from build123d import *

# Parameters (mm, degrees)
EXTRU_MINCE1_DEPTH         = 100
EXTRU_MINCE2_DEPTH         = 5
EXTRU_MINCE3_DEPTH         = 5
CONG_1_R                   = 10
R_P_TITION_START           = 80
R_P_TITION_LIN_AIRE1_DEPTH = 5
CONG_2_R                   = 5


# Read off the part's stored shape, not the designer's step: Répétition linéaire1
with BuildPart() as part:
    # Esquisse1 → Extru.-Mince1 (new body)
    with BuildSketch(Plane.XY):
        Polygon((0, 0), (-65.404068622, 0), (-4.782306964, 200), (-0.954292763, 198.839695178), (-60.011920576, 4), (0, 4), align=None)
    extrude(amount=EXTRU_MINCE1_DEPTH)

    # Esquisse2 → Extru.-Mince2 (add)
    with BuildSketch(Plane.XY.offset(10)):
        Polygon((-11.060818094, 179.286279518), (-14.23934022, 192.904801434), (-10.344030265, 193.813955082), (-7.16550814, 180.195433166), align=None)
        Polygon((-40.068438655, 83.585924506), (-43.246960781, 97.204446422), (-39.351650826, 98.11360007), (-36.1731287, 84.495078154), align=None)
    extrude(amount=EXTRU_MINCE2_DEPTH)

    # Esquisse3 → Extru.-Mince3 (add)
    with BuildSketch(Plane.XY.offset(45)):
        Polygon((-18.341466727, 155.266361808), (-26.702263311, 169.885700914), (-23.229995746, 171.871489915), (-14.869199162, 157.252150809), align=None)
        Polygon((-32.333054107, 109.106082076), (-40.693850691, 123.725421182), (-37.221583126, 125.711210183), (-28.860786542, 111.091871077), align=None)
        Polygon((-51.073031786, 47.280172809), (-59.433828371, 61.899511915), (-55.961560806, 63.885300916), (-47.600764221, 49.26596181), align=None)
    extrude(amount=EXTRU_MINCE3_DEPTH)

    # Congé1
    cong_1_edges = [part.edges().sort_by_distance(p)[0] for p in [
        (-11.060818094, 179.286279518, 12.5),
        (-40.068438655, 83.585924506, 12.5),
        (-18.341466727, 155.266361808, 47.5),
        (-32.333054107, 109.106082076, 47.5),
        (-51.073031786, 47.280172809, 47.5),
    ]]
    fillet(cong_1_edges, radius=CONG_1_R)

    # Répétition linéaire1 outline → Répétition linéaire1 (add)
    with BuildSketch(Plane.XY.offset(R_P_TITION_START)):
        with BuildLine():
            Line((-40.845695505, 81.021641222), (-37.74782901, 91.241952907))
            Line((-37.74782901, 91.241952907), (-39.351650826, 98.11360007))
            Line((-39.351650826, 98.11360007), (-43.246960781, 97.204446422))
            Line((-43.246960781, 97.204446422), (-40.677456119, 86.195287398))
            ThreePointArc((-40.677456119, 86.195287398), (-40.421014092, 83.597389742), (-40.845695505, 81.021641222))
        make_face()
        with BuildLine():
            Line((-8.74020845, 186.942307919), (-10.344030265, 193.813955082))
            Line((-10.344030265, 193.813955082), (-14.23934022, 192.904801434))
            Line((-14.23934022, 192.904801434), (-11.669835559, 181.89564241))
            ThreePointArc((-11.669835559, 181.89564241), (-11.413393531, 179.297744754), (-11.838074945, 176.721996234))
            Line((-11.838074945, 176.721996234), (-8.74020845, 186.942307919))
        make_face()
    extrude(amount=R_P_TITION_LIN_AIRE1_DEPTH)

    # Congé2
    cong_2_edges = [part.edges().sort_by_distance(p)[0] for p in [
        (0, 2, 100),
        (0, 2, 0),
        (-2.868299864, 199.419847589, 0),
        (-2.868299864, 199.419847589, 100),
        (-60.011920576, 4, 50),
        (-65.404068622, 0, 50),
    ]]
    fillet(cong_2_edges, radius=CONG_2_R)


solid = part.part
Source: CAD feature listing. Evaluate the final solid. Frame: model axes, mm. A direction names the side the tool comes from. Give positions to 0.01 mm unless a question says otherwise; leave off trailing zeros. Write each loop counter-clockwise with the first axis right and the second up, starting at its lowest first coordinate (ties: lowest second). Pieces come first, ordered by that corner, then holes. Notation, with made-up numbers: (52.25, 26) - (60.25, 26) arc R18 ccw to (60.25, 46) - close; hole circle Ø10 at (39, 39.5). An arc over 180 degrees is marked (long way). Write item = value, one per line. Start each with the question number.
Q1. Draft query along Z for faces 1 (the flat face through (-33, 98, 0)), 2 (the flat face through (-12, 187, 85)), 3 (the flat face through (-12.319, 193.353, 12.465)), 4 (the flat face through (-12, 187, 80)). Return one class per face: +Z half, -Z half, draft (parallel to the pull), parting line (faces both ways), or undercut.
Q2. Material intervals for probe 1 along X at (y, z) = (116.5, 69); probe 2 along X at (y, z) = (175.5, 31), sorted ascending.
Q3. Cut plane A-A, the plane y = 165.5. Return loops of the section in (x, z).
Q4. Reachability of faces 5 (the flat face through (-41, 92, 80)), 6 (the cylindrical face through (-2, 2, 99)), 7 (the flat face through (-40, 93, 10)) from +Z, -Z, +X, -X, +Y, -Y: full face, straight path, thin tool, end or side. Return the list, or none.
Q5. Cut plane C-C, the plane y = 73.5. Return loops of the section in (x, z).
Q6. Cut plane B-B, the plane z = 35.5. Return loops of the section in (x, y), then the cut area to 3 significant figures.
Q7. Pin query (flat end, axial travel): pin 1 Ø2.5 at (x, y) = (-12, 182) entering from +Z; pin 2 Ø3 at (x, y) = (-23, 166) entering from +Z; pin 3 Ø5 at (x, y) = (-37, 115) entering from -Z. Return the tip coordinate at first contact, or that it passes through.
Computed values:
q1.face_1 = -Z half
q1.face_2 = +Z half
q1.face_3 = draft
q1.face_4 = undercut
q2.probe_1 = -30.09 to -25.91
q2.probe_2 = -12.21 to -8.03
q3.outline = (-24.19, 45) - (-19.59, 45) - (-19.59, 50) - (-24.19, 50) - close; (-15.24, 0) - (-11.06, 0) - (-11.06, 100) - (-15.24, 100) - close
q4.face_5 = -X, +Y
q4.face_6 = +Z, +X, -Y
q4.face_7 = -Z, -X, +Y
q5.outline = (-43.13, 0) - (-38.95, 0) - (-38.95, 100) - (-43.13, 100) - close
q6.outline = (-63.45, 6.45) arc R5 ccw to (-58.66, 0) - (0, 0) - (0, 4) - (-53.27, 4) arc R5 cw to (-58.06, 10.45) - (-0.95, 198.84) - (-4.78, 200) - close
q6.area = 1,080 mm²
q7.pin_1 = 85
q7.pin_2 = 50
q7.pin_3 = 45
